Autodesk Inventor part; units mm, degrees
ref_plane "YZ Plane" through (0, 0, 0) normal (1, 0, 0) x (0, 1, 0)
ref_plane "XZ Plane" through (0, 0, 0) normal (0, 1, 0) x (-1, 0, 0)
ref_plane "XY Plane" through (0, 0, 0) normal (0, 0, 1) x (1, 0, 0)
sketch "Sketch1" plane through (0, 0, 0) normal (0, 0, 1) x (1, 0, 0)
  line L0 (-41.5, 50) -> (41.5, 50)
  line L1 (41.5, 50) -> (41.5, -50)
  line L2 (41.5, -50) -> (-41.5, -50)
  line L3 (-41.5, -50) -> (-41.5, 50)
  line L4 (31.5, 40) -> (-31.5, 40)
  line L5 (-31.5, 40) -> (-31.5, -40)
  line L6 (-31.5, -40) -> (31.5, -40)
  line L7 (31.5, -40) -> (31.5, 40)
  line L8 (-41.5, -45) -> (41.5, -45) construction
  line L9 (0, 71.7466) -> (0, -78.0681) construction
  line L10 (-60.2597, 0) -> (74.2823, 0) construction
  line L11 (-36.5, 50) -> (-36.5, -50) construction
  circle A0 centre (-36.5, -27) radius 2.25
  line L12 (-41.5, 45) -> (41.5, 45) construction
  circle A1 centre (-36.5, 45) radius 2.25
  circle A2 centre (-36.5, -45) radius 2.25
  circle A3 centre (-36.5, 27) radius 2.25
  circle A4 centre (-25, -45) radius 2.25
  circle A5 centre (25, -45) radius 2.25
  line L13 (30, 50) -> (30, -50) construction
  line L14 (-30, 50) -> (-30, -50) construction
  line L15 (-31, -38) -> (31, -38)
  line L16 (31, -38) -> (31, -52)
  line L17 (31, -52) -> (-31, -52)
  line L18 (-31, -52) -> (-31, -38)
  line L19 (-31.5, -40) -> (-16.5, -40)
  line L20 (-16.5, -40) -> (-16.5, -20)
  line L21 (-16.5, -20) -> (-31.5, -20)
  line L22 (-31.5, -20) -> (-31.5, -40)
  line L23 (-26.5, -26) -> (-21.5, -26) construction
  line L24 (-26.5, -27.5) -> (-21.5, -27.5)
  line L25 (-21.5, -24.5) -> (-26.5, -24.5)
  arc A6 (-26.5, -24.5) -> (-26.5, -27.5) centre (-26.5, -26) ccw
  arc A7 (-21.5, -27.5) -> (-21.5, -24.5) centre (-21.5, -26) ccw
  line L26 (-26.5, -34) -> (-21.5, -34) construction
  line L27 (-26.5, -35.5) -> (-21.5, -35.5)
  line L28 (-21.5, -32.5) -> (-26.5, -32.5)
  arc A8 (-26.5, -32.5) -> (-26.5, -35.5) centre (-26.5, -34) ccw
  arc A9 (-21.5, -35.5) -> (-21.5, -32.5) centre (-21.5, -34) ccw
  line L29 (-43.5, 33) -> (-29.5, 33)
  line L30 (-29.5, 33) -> (-29.5, -33)
  line L31 (-29.5, -33) -> (-43.5, -33)
  line L32 (-43.5, -33) -> (-43.5, 33)
  point P0 (0, 0)
  point P1 (0, 50)
  point P2 (41.5, 0)
  point P3 (0, 45)
  point P4 (-24, -26)
  point P5 (-24, -20)
  point P6 (-16.5, -30)
  point P7 (-24, -34)
  dimension "d0" = 83
  dimension "d1" = 100
  dimension "d5" = 5
  dimension "d6" = 5
  dimension "d9" = 5
  dimension "d12" = 4.5
  dimension "d17" = 5
  dimension "d41" = 4.5
  dimension "d42" = 4.5
  dimension "d87" = 4.5
  dimension "d89" = 4.5
  dimension "d90" = 4.5
  dimension "d91" = 30
  dimension "d92" = 30
  dimension "d93" = 5
  dimension "d94" = 5
  dimension "d97" = 1
  dimension "d98" = 2
  dimension "d99" = 2
  dimension "d100" = 1
  dimension "d103" = 15
  dimension "d104" = 20
  dimension "d105" = 5
  dimension "d106" = 3
  dimension "d109" = 5
  dimension "d110" = 3
  dimension "d112" = 6
  dimension "d113" = 6
  dimension "d115" = 6
  dimension "d116" = 2
  dimension "d117" = 2
  dimension "d118" = 6
  dimension "d121" = 27
  dimension "d122" = 27
extrude "Extrusion12" add sketch "Sketch1" along normal blind 1.5 contours L0 L1 L2 L16 L6 L7 L4 L5 L29 L3 | L29 L5 L31 L3 | L31 L5 L6 L18 L2 L3 | L2 L18 L6 L16 | A0 | A1 | A2 | A3 | A4 | A5
extrude "Extrusion13" cut sketch "Sketch1" along normal blind 1.5 contours A0 | A1 | A2 | A3
extrude "Extrusion14" cut sketch "Sketch1" along normal blind 1.5 contours A4 | A5
mirror "Mirror6" about plane through (0, 0, 0) normal (0, 1, 0) of "Extrusion14"
mirror "Mirror7" about plane through (0, 0, 0) normal (1, 0, 0) of "Extrusion13"
equation "\"d12\" = screw"
equation "\"d41\" = screw"
equation "\"d42\" = screw"
equation "\"d87\" = screw"
equation "\"d89\" = screw"
equation "\"d90\" = screw"
properties part number "Side" material "PC/ABS Plastic"
Could you check a few things on this model? Use its own coordinates, in mm. Give positions to 0.01 mm unless a question says otherwise; leave off trailing zeros. Loops run counter-clockwise (first coordinate to the right, second up) from the corner with the lowest first, then second, coordinate; pieces in that order, holes last. Notation, with made-up numbers: (62.5, 30.5) - (81.5, 30.5) arc R9 ccw to (81.5, 47.5) - close; hole circle Ø3 at (79.25, -16.75). An arc over 180 degrees is marked (long way). Answer in a Markdown table with one row per item. Add a question column.
Q1. We'd pull the mould along X, two halves only. Please class faces 1 (the face through (-35.29, -46.897, 0.74)), 2 (the face through (-34, 4, 0)): +X half, -X half, draft (parallel to the pull), parting line (faces both ways), or undercut.
Q2. For pin 1 (7 mm diameter, centred on x = 25, y = 45, fed in from -Z), with a flat end and sliding along its axis, tell me the tip position at first contact or that it passes through.
Q3. If we section it at A-A (x = 36.5): List the corners of the cut face in (y, z) for me.
Q4. If we section it at B-B (y = -45): List the corners of the cut face in (x, z) for me, plus the area to 3 significant figures.
Q5. Please list where these lines run through material, in increasing order: L1, parallel to Y at x = 36.5, z = 0.75; L2, parallel to Y at x = 25, z = 0.7; L3, parallel to Y at x = -10, z = 0.3. Write a range as from..to.
Q6. If we section it at D-D (y = 10): List the corners of the cut face in (x, z) for me.
Q7. If we section it at C-C (z = 0.25): State how many separate pieces and enclosed holes the cut face has, plus the area to 3 significant figures.
The answers:
| question | item | result |
|---|---|---|
| 1 | face 1 | undercut |
| 1 | face 2 | draft |
| 2 | pin 1 | stops at z = 0 |
| 3 | outline | (-50, 0) - (-47.25, 0) - (-47.25, 1.5) - (-50, 1.5) - close; (-42.75, 0) - (-29.25, 0) - (-29.25, 1.5) - (-42.75, 1.5) - close; (-24.75, 0) - (24.75, 0) - (24.75, 1.5) - (-24.75, 1.5) - close; (29.25, 0) - (42.75, 0) - (42.75, 1.5) - (29.25, 1.5) - close; (47.25, 0) - (50, 0) - (50, 1.5) - (47.25, 1.5) - close |
| 4 | outline | (-41.5, 0) - (-38.75, 0) - (-38.75, 1.5) - (-41.5, 1.5) - close; (-34.25, 0) - (-27.25, 0) - (-27.25, 1.5) - (-34.25, 1.5) - close; (-22.75, 0) - (22.75, 0) - (22.75, 1.5) - (-22.75, 1.5) - close; (27.25, 0) - (34.25, 0) - (34.25, 1.5) - (27.25, 1.5) - close; (38.75, 0) - (41.5, 0) - (41.5, 1.5) - (38.75, 1.5) - close |
| 4 | area | 97.5 mm^2 |
| 5 | L1 | y = -50..-47.25, -42.75..-29.25, -24.75..24.75, 29.25..42.75, 47.25..50 |
| 5 | L2 | y = -50..-47.25, -42.75..-40, 40..42.75, 47.25..50 |
| 5 | L3 | y = -50..-40, 40..50 |
| 6 | outline | (-41.5, 0) - (-31.5, 0) - (-31.5, 1.5) - (-41.5, 1.5) - close; (31.5, 0) - (41.5, 0) - (41.5, 1.5) - (31.5, 1.5) - close |
| 7 | separate pieces | 1 |
| 7 | enclosed holes | 13 |
| 7 | area | 3,070 mm^2 |
